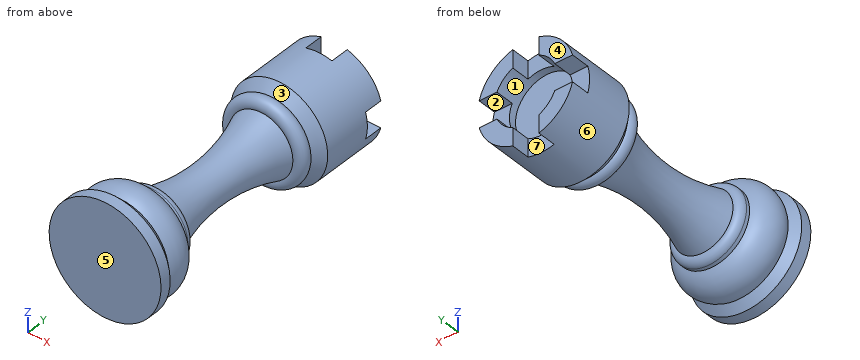
```python
from build123d import *

# Parameters (mm, degrees)
CUT_EXTRUDE1_DEPTH = 5
CIRPATTERN1_COUNT  = 4


with BuildPart() as part:
    # Sketch1 → Revolve2 (revolve)
    with BuildSketch(Plane.XY, mode=Mode.PRIVATE) as revolve2_sk:
        with BuildLine():
            Line((0, 0), (-15, 0))
            Line((-15, 0), (-15, 3))
            Line((-15, 3), (-13, 5))
            ThreePointArc((-13, 5), (-13.688325627, 10.216881481), (-10, 13.97))
            Line((-10, 13.97), (-10, 14.97))
            ThreePointArc((-10, 14.97), (-9.414213562, 16.384213562), (-8, 16.97))
            ThreePointArc((-8, 16.97), (-5.234654729, 34.114083995), (-8.5, 51.17))
            ThreePointArc((-8.5, 51.17), (-11, 52.00581604), (-10.5, 54.593979182))
            Line((-10.5, 54.593979182), (-13, 57.093979182))
            Line((-13, 57.093979182), (-13, 75.093979182))
            Line((-13, 75.093979182), (-8.5, 75.093979182))
            Line((-8.5, 75.093979182), (-8.5, 68.093979182))
            Line((-8.5, 68.093979182), (0, 68.093979182))
            Line((0, 68.093979182), (0, 0))
        make_face()
    revolve(revolve2_sk.sketch.rotate(Axis((0, 75.093979182, 0), (0, -1, 0)), 270), axis=Axis((0, 75.093979182, 0), (0, -1, 0)))

    # Sketch2 → Cut-Extrude1 (cut)
    with BuildSketch(Plane(origin=(0, 75.093979182, 0), x_dir=(1, 0, 0), z_dir=(0, 1, 0))):
        with BuildLine():
            ThreePointArc((8.5, 0), (8.309353672, -1.790151267), (7.745966692, -3.5))
            Line((7.745966692, -3.5), (12.519984026, -3.5))
            ThreePointArc((12.519984026, -3.5), (12.879436951, -1.766381565), (13, 0))
            ThreePointArc((13, 0), (12.879436951, 1.766381565), (12.519984026, 3.5))
            Line((12.519984026, 3.5), (7.745966692, 3.5))
            ThreePointArc((7.745966692, 3.5), (8.309353672, 1.790151267), (8.5, 0))
        make_face()
    cut_extrude1 = extrude(amount=-CUT_EXTRUDE1_DEPTH, mode=Mode.SUBTRACT)

    # CirPattern1: Cut-Extrude1 ×4 about axis
    cirpattern1_axis = Axis((0, 0, 0), (0, 1, 0))
    for i in range(1, CIRPATTERN1_COUNT):
        add(cut_extrude1.rotate(cirpattern1_axis, i * 360 / CIRPATTERN1_COUNT), mode=Mode.SUBTRACT)


solid = part.part
```
Part model, mm, in its own coordinate system. Face numbers are marked on the shaded views. A direction names the side the tool comes from. Give positions to 0.01 mm unless a question says otherwise; leave off trailing zeros. Loops run counter-clockwise (first coordinate to the right, second up) from the corner with the lowest first, then second, coordinate; pieces in that order, holes last. Notation, with made-up numbers: M 10,76.25 L 65,76.25 A36 cw 65,110.25 Z; hole C -23,15.25 d8. An arc over 180 degrees is marked long. Return JSON: item names as keys, results as strings.
1) Pull direction X, two halves, no side cores. Call the marked faces 5, 6 and 7: released by +X, released by -X, zero draft, split by the parting line, or undercut.
Calculated:
{"face 5": "zero draft", "face 6": "split by the parting line", "face 7": "undercut"}
2) Saw through at C-C, the plane y = 10. List the corners of the cut face in (x, z).
Calculated:
{"outline": "C 0,0 d27.51"}
3) Saw through at B-B, the plane y = 66. List the corners of the cut face in (x, z).
Calculated:
{"outline": "C 0,0 d26"}
4) Drill centre lines: line 1 (X direction, y = 70, z = 0); line 2 (Y direction, x = -4.25, z = 11.5); line 3 (Y direction, x = -7.25, z = 6.5). Where is each one in solid material? Low to high.
Calculated:
{"line 1": "x = -13 to -8.5, 8.5 to 13", "line 2": "y = 0 to 12.54, 56.35 to 75.09", "line 3": "y = 0 to 15.96, 51.07 to 75.09"}
5) Flat gauge pins, fed straight in: pin 1 Ø5.5 at (y, z) = (71.5, 9) entering from -X; pin 2 Ø2.5 at (y, z) = (71.5, -10) entering from +X; pin 3 Ø2.5 at (x, z) = (-11, 1) entering from +Y. Where does each tip first touch, or does it go through?
Calculated:
{"pin 1": "stops at x = -11.4", "pin 2": "stops at x = 9.61", "pin 3": "stops at y = 70.09"}
6) 3-axis set-ups, long thin cutter, end or side, ignore diameter. For the marked faces 1, 2, 3 and 4: which of +Z, -Z, +X, -X, +Y, -Y reach the whole face in a straight line?
Calculated:
{"face 1": "+Y", "face 2": "+X, -X, +Y", "face 3": "none", "face 4": "+Z, -Z, +X, -X, +Y"}
7) Saw through at A-A, the plane x = 0. List the corners of the cut face in (y, z).
Calculated:
{"outline": "M 0,-15 L 3,-15 L 5,-13 A6 ccw 13.97,-10 L 14.97,-10 A2 ccw 16.97,-8 A50 cw 51.17,-8.5 A2 ccw 54.59,-10.5 L 57.09,-13 L 70.09,-13 L 70.09,-8.5 L 68.09,-8.5 L 68.09,8.5 L 70.09,8.5 L 70.09,13 L 57.09,13 L 54.59,10.5 A2 ccw 51.17,8.5 A50 cw 16.97,8 A2 ccw 14.97,10 L 13.97,10 A6 ccw 5,13 L 3,15 L 0,15 Z"}
